Can you work these out from the model? Positions are in its coordinate system, mm. A direction names the side the tool comes from. Give positions to 0.01 mm unless a question says otherwise; leave off trailing zeros. Write each loop counter-clockwise with the first axis right and the second up, starting at its lowest first coordinate (ties: lowest second). Pieces come first, ordered by that corner, then holes.
1. Suppose I cut it at B-B (z = 30). Please give me the cut outline in (x, y).
2. Suppose I cut it at A-A (z = 15). Please give me the cut outline in (x, y).
3. Suppose I cut it at D-D (x = 32.5). Please give me the cut outline in (y, z), and give its area (3 significant figures).
4. On a 3-axis mill with a long thin cutter (end or side, diameter ignored), from which of +Z, -Z, +X, -X, +Y, -Y can I reach the whole of each face in a straight line? I mean faces 4 (the flat face through (25, 5, 24)), 5 (the cylindrical face through (27.48, 2.54, 29.67)). Say none if no direction works.
5. If I drill on probe 1 along Y at (x, z) = (40, 1.85); probe 2 along X at (y, z) = (2.7, 45); probe 3 along X at (y, z) = (3, 30), over which ranges is the centre line in solid material (lowest first)?
6. I'm going to push flat-ended pins straight in: pin 1 (8 mm diameter, centred on x = 40, z = 45, fed in from +Y); pin 2 (6 mm diameter, centred on x = 7.5, y = 29.5, fed in from +Z). Where does each tip first touch, or does it pass through?
7. Suppose I cut it at C-C (y = 31.5). Please give me the cut outline in (x, z), and give its area (3 significant figures).
8. Thinking about a two-plate mould opening in Y: for faces 1 (the cylindrical face through (2.85, 2.54, 51.99)), 2 (the cylindrical face through (9.46, 12.56, 2.54)), 3 (the cylindrical face through (46.99, 32.15, 2.46)), which applies, pulls with the +Y half, pulls with the -Y half, needs draft (parallel to the pull), parting line crosses it, or undercut?
```python
from build123d import *

# Parameters (mm, degrees)
SKETCH1_W           = 50
SKETCH1_H           = 60
BOSS_EXTRUDE1_DEPTH = 5
SKETCH2_W           = 50
SKETCH2_H           = 5
BOSS_EXTRUDE2_DEPTH = 50
SKETCH3_W           = 50
SKETCH3_H           = 5
CUT_EXTRUDE1_DEPTH  = 5
SKETCH4_R           = 2.5
CUT_EXTRUDE2_DEPTH  = 5
SKETCH5_R           = 2.5
CUT_EXTRUDE3_DEPTH  = 5
FILLET1_R           = 10
SKETCH7_W           = 50
SKETCH7_H           = 5
CUT_EXTRUDE4_DEPTH  = 20
FILLET2_R           = 10
SKETCH8_R           = 2.5
CUT_EXTRUDE5_DEPTH  = 20
SKETCH9_R           = 2.5
BOSS_EXTRUDE3_DEPTH = 5


with BuildPart() as part:
    # Sketch1 → Boss-Extrude1 (new body)
    with BuildSketch(Plane.XY):
        with Locations((25, 30)):
            Rectangle(SKETCH1_W, SKETCH1_H)
    extrude(amount=BOSS_EXTRUDE1_DEPTH)

    # Sketch2 → Boss-Extrude2 (add)
    with BuildSketch(Plane.XY.offset(5)):
        with Locations((25, 2.5)):
            Rectangle(SKETCH2_W, SKETCH2_H)
    extrude(amount=BOSS_EXTRUDE2_DEPTH)

    # Sketch3 → Cut-Extrude1 (cut)
    with BuildSketch(Plane(origin=(0, 60, 0), x_dir=(1, 0, 0), z_dir=(0, 1, 0))):
        with Locations((25, -2.5)):
            Rectangle(SKETCH3_W, SKETCH3_H)
    extrude(amount=-CUT_EXTRUDE1_DEPTH, mode=Mode.SUBTRACT)

    # Sketch4 → Cut-Extrude2 (cut)
    with BuildSketch(Plane(origin=(0, 5, 0), x_dir=(1, 0, 0), z_dir=(0, 1, 0))):
        with Locations(Location((10, -15, 0), (0, 0, 270))):
            Circle(SKETCH4_R)
        with Locations(Location((25, -30, 0), (0, 0, 270))):
            Circle(SKETCH4_R)
        with Locations(Location((40, -15, 0), (0, 0, 270))):
            Circle(SKETCH4_R)
        with Locations(Location((40, -45, 0), (0, 0, 270))):
            Circle(SKETCH4_R)
        with Locations(Location((10, -45, 0), (0, 0, 270))):
            Circle(SKETCH4_R)
    extrude(amount=-CUT_EXTRUDE2_DEPTH, mode=Mode.SUBTRACT)

    # Sketch5 → Cut-Extrude3 (cut)
    with BuildSketch(Plane.XY.offset(5)):
        with Locations((10, 45)):
            Circle(SKETCH5_R)
        with Locations((25, 30)):
            Circle(SKETCH5_R)
        with Locations((40, 45)):
            Circle(SKETCH5_R)
        with Locations((40, 15)):
            Circle(SKETCH5_R)
        with Locations((10, 15)):
            Circle(SKETCH5_R)
    extrude(amount=-CUT_EXTRUDE3_DEPTH, mode=Mode.SUBTRACT)

    # Fillet1
    fillet1_edges = [part.edges().sort_by_distance(p)[0] for p in [
        (50, 55, 2.5),
        (0, 55, 2.5),
        (0, 2.5, 55),
        (50, 2.5, 55),
    ]]
    fillet(fillet1_edges, radius=FILLET1_R)

    # Sketch7 → Cut-Extrude4 (cut)
    with BuildSketch(Plane(origin=(0, 55, 0), x_dir=(1, 0, 0), z_dir=(0, 1, 0))):
        with Locations((25, -2.5)):
            Rectangle(SKETCH7_W, SKETCH7_H)
    extrude(amount=-CUT_EXTRUDE4_DEPTH, mode=Mode.SUBTRACT)

    # Fillet2
    fillet2_edges = [part.edges().sort_by_distance(p)[0] for p in [
        (50, 35, 2.5),
        (0, 35, 2.5),
    ]]
    fillet(fillet2_edges, radius=FILLET2_R)

    # Sketch8 → Cut-Extrude5 (cut)
    with BuildSketch(Plane.XY.offset(5)):
        with Locations((10, 30)):
            Circle(SKETCH8_R)
        with Locations((40, 30)):
            Circle(SKETCH8_R)
    extrude(amount=-CUT_EXTRUDE5_DEPTH, mode=Mode.SUBTRACT)

    # Sketch9 → Boss-Extrude3 (add, through all)
    with BuildSketch(Plane.XY.offset(5)):
        with Locations((25, 30)):
            Circle(SKETCH9_R)
    extrude(amount=-BOSS_EXTRUDE3_DEPTH)


solid = part.part
```
Checks:
1. outline: (0, 0) - (22.5, 0) - (22.5, 5) - (0, 5) - close; (27.5, 0) - (50, 0) - (50, 5) - (27.5, 5) - close
2. outline: (0, 0) - (7.5, 0) - (7.5, 5) - (0, 5) - close; (12.5, 0) - (37.5, 0) - (37.5, 5) - (12.5, 5) - close; (42.5, 0) - (50, 0) - (50, 5) - (42.5, 5) - close
3. outline: (0, 0) - (35, 0) - (35, 5) - (5, 5) - (5, 55) - (0, 55) - close
3. area: 425 mm2
4. face 4: +Z, +X, -X, +Y
4. face 5: +Y, -Y
5. probe 1: y = 0 to 12.5, 17.5 to 27.5, 32.5 to 35
5. probe 2: x = 0 to 7.5, 12.5 to 37.5, 42.5 to 50
5. probe 3: x = 0 to 22.5, 27.5 to 50
6. pin 1: stops at y = 5
6. pin 2: stops at z = 5
7. outline: (2.4, 0) - (8, 0) - (8, 5) - (2.4, 5) - close; (12, 0) - (38, 0) - (38, 5) - (12, 5) - close; (42, 0) - (47.6, 0) - (47.6, 5) - (42, 5) - close
7. area: 186 mm2
8. face 1: needs draft
8. face 2: undercut
8. face 3: pulls with the +Y half
